from build123d import *

# Parameters (mm, degrees)
F0_W     = 18
F0_H     = 18
F1_DEPTH = 25
F2_W     = 12.4
F2_H     = 12.4
F3_DEPTH = 4
F4_W     = 15
F4_H     = 15
F5_DEPTH = 15
F6_W     = 10.6
F6_H     = 10.6
F7_DEPTH = 11
F8_R     = 1


with BuildPart() as f1:
    # F0 (on Top) → F1 (new body)
    with BuildSketch(Plane.XY):
        Rectangle(F0_W, F0_H)
    extrude(amount=F1_DEPTH)

    # F2 (on face) → F3 (join)
    with BuildSketch(Plane.XY.offset(25)):
        Rectangle(F2_W, F2_H)
    extrude(amount=F3_DEPTH)

    # F4 (on face) → F5 (cut)
    with BuildSketch(Plane(origin=(0, 0, 0), x_dir=(1, 0, 0), z_dir=(0, 0, -1))):
        Rectangle(F4_W, F4_H)
    extrude(amount=-F5_DEPTH, mode=Mode.SUBTRACT)

    # F6 (on face) → F7 (cut)
    with BuildSketch(Plane(origin=(0, 0, 15), x_dir=(1, 0, 0), z_dir=(0, 0, -1))):
        Rectangle(F6_W, F6_H)
    extrude(amount=-F7_DEPTH, mode=Mode.SUBTRACT)

    # F8
    f8_edges = [f1.edges().sort_by_distance(p)[0] for p in [
        (6.2, -6.2, 27),
        (6.2, 6.2, 27),
        (-6.2, 6.2, 27),
        (-6.2, -6.2, 27),
    ]]
    fillet(f8_edges, radius=F8_R)


solid = f1.part
Could you check a few things on this model? Use its own coordinates, in mm. A direction names the side the tool comes from. Give positions to 0.01 mm unless a question says otherwise; leave off trailing zeros. Write each loop counter-clockwise with the first axis right and the second up, starting at its lowest first coordinate (ties: lowest second). Pieces come first, ordered by that corner, then holes. Notation, with made-up numbers: (80, 84) -> (138, 84) arc R17 ccw to (138, 101) -> close; hole circle Ø1 at (77, 47). An arc over 180 degrees is marked (long way). Write each question's results on one line, items separated by ' | '. Start each with the question number.
Q1. Which directions (+Z, -Z, +X, -X, +Y, -Y) give clear straight access to the entire face, cutting with the end or side of a thin tool? Please do faces 1 (the face through (0, -6.2, 27)), 2 (the face through (-8, 0, 25)), 3 (the face through (-5.899, -5.915, 27.028)), 4 (the face through (0, 0, 26)).
Q2. I'm going to push flat-ended pins straight in: pin 1 Ø6 at (x, y) = (-4, -3.5) entering from -Z; pin 2 Ø3 at (y, z) = (0.5, 27) entering from +X; pin 3 Ø3 at (y, z) = (-1, 26) entering from -X. Where does each tip first touch, or does it pass through?
Q3. Suppose I cut it at B-B, the plane y = 2.5. List the corners of the cut face in (x, z) for me, and give its area (3 significant figures).
Q4. Suppose I cut it at C-C, the plane z = 26.75. List the corners of the cut face in (x, y) for me.
Q5. Suppose I cut it at A-A, the plane z = 11.75. List the corners of the cut face in (x, y) for me, and give its area (3 significant figures).
Q6. I need wall thicknesses on probe 1 along Y at (x, z) = (-5, 3.5); probe 2 along Y at (x, z) = (-5.25, 18.75). Which ranges of each line are inside material? Lowest first, please.
Q7. We'd pull the mould along Y, two halves only. Please class faces 5 (the face through (7.5, 0, 7)), 6 (the face through (-6.2, 0, 27)), 7 (the face through (-5.899, 5.915, 27.028)): +Y half, -Y half, draft (parallel to the pull), parting line (faces both ways), or undercut.
Outcome:
1) face 1: +Z, +X, -X, -Y | face 2: +Z | face 3: +Z, -X, -Y | face 4: -Z
2) pin 1: z = 15 | pin 2: x = 6.2 | pin 3: x = -9
3) outline: (-9, 0) -> (-7.5, 0) -> (-7.5, 15) -> (-5.3, 15) -> (-5.3, 26) -> (5.3, 26) -> (5.3, 15) -> (7.5, 15) -> (7.5, 0) -> (9, 0) -> (9, 25) -> (6.2, 25) -> (6.2, 29) -> (-6.2, 29) -> (-6.2, 25) -> (-9, 25) -> close | area: 158 mm2
4) outline: (-6.2, -5.2) arc R1 ccw to (-5.2, -6.2) -> (5.2, -6.2) arc R1 ccw to (6.2, -5.2) -> (6.2, 5.2) arc R1 ccw to (5.2, 6.2) -> (-5.2, 6.2) arc R1 ccw to (-6.2, 5.2) -> close
5) outline: (-9, -9) -> (9, -9) -> (9, 9) -> (-9, 9) -> close; hole (-7.5, -7.5) -> (7.5, -7.5) -> (7.5, 7.5) -> (-7.5, 7.5) -> close | area: 99.0 mm2
6) probe 1: -9 to -7.5, 7.5 to 9 | probe 2: -9 to -5.3, 5.3 to 9
7) face 5: undercut | face 6: draft | face 7: +Y half
